Read the model definition and answer for the solid it produces. Units are mm, in the model's axes. Coordinates: 2 decimals unless noted, no trailing zeros. Loops run counter-clockwise (first coordinate to the right, second up) from the corner with the lowest first, then second, coordinate; pieces in that order, holes last. Notation, with made-up numbers: M 24.25,18.25 L 30.25,18.25 A22 cw 30.25,37.25 Z; hole C 27.25,-0.5 d11. An arc over 180 degrees is marked long. One line per item, written item: value. Start each with the question number.
1. The part is cut by section C-C (y = -21.5). Write down the section's boundary in (x, z).
2. Determine the mould class of faces 1 (the face through (-16, -41, 0)), 2 (the face through (-14.276, 47, 3)), 3 (the face through (-1, -62.803, 3)), 4 (the face through (-56.78, 56.76, 3.22)) for opening direction Y: +Y half, -Y half, draft (parallel to the pull), parting line (faces both ways), or undercut.
3. A flat-ended cylindrical pin translates along its axis: pin 1 (6.5 mm diameter, centred on x = -55.9, y = -53.99, fed in from +Z). Find the tip coordinate at first contact, or state that the pin passes through.
4. The part is cut by section D-D (z = 4.5). State how many separate pieces and enclosed holes the cut face has, then the cut area to 3 significant figures.
5. Consider probe 1 along Y at (x, z) = (57, 2); probe 2 along X at (y, z) = (-16.5, 0.5); probe 3 along Y at (x, z) = (-4.5, 3.75). Determine where each line is inside the solid, lowest interval first.
6. The part is cut by section A-A (x = 27). Write down the section's boundary in (y, z), then the cut area to 3 significant figures.
7. The part is cut by section B-B (x = 58). Write down the section's boundary in (y, z), then the cut area to 3 significant figures.
```python
from build123d import *

# Parameters (mm, degrees)
SKETCH2_W           = 132.7
SKETCH2_H           = 125
BOSS_EXTRUDE1_DEPTH = 6.35
SKETCH1_R           = 2
CUT_EXTRUDE1_DEPTH  = 6.35
SKETCH6_R           = 4
CUT_EXTRUDE3_DEPTH  = 6.35


with BuildPart() as part:
    # Sketch2 → Boss-Extrude1 (new body)
    with BuildSketch(Plane.XY):
        with Locations((-0.075710713, -0.302842853)):
            Rectangle(SKETCH2_W, SKETCH2_H)
    extrude(amount=BOSS_EXTRUDE1_DEPTH)

    # Sketch1 → Cut-Extrude1 (cut)
    with BuildSketch(Plane.XY):
        with Locations(Location((-50.481706077, 16.075057848, 0), (0, 0, 180))):
            Circle(SKETCH1_R)
        with Locations(Location((-50.481706077, -16.680743555, 0), (0, 0, 180))):
            Circle(SKETCH1_R)
        with Locations(Location((-31.228329085, -43.180743555, 0), (0, 0, 180))):
            Circle(SKETCH1_R)
        with Locations(Location((-0.075710713, -53.302842853, 0), (0, 0, 180))):
            Circle(SKETCH1_R)
        with Locations(Location((31.076907658, -43.180743555, 0), (0, 0, 180))):
            Circle(SKETCH1_R)
        with Locations(Location((50.33028465, -16.680743555, 0), (0, 0, 180))):
            Circle(SKETCH1_R)
        with Locations(Location((50.33028465, 16.075057848, 0), (0, 0, 180))):
            Circle(SKETCH1_R)
        with Locations(Location((31.076907658, 42.575057848, 0), (0, 0, 180))):
            Circle(SKETCH1_R)
        with Locations(Location((-31.228329085, 42.575057848, 0), (0, 0, 180))):
            Circle(SKETCH1_R)
        with BuildLine():
            Line((-14.275710713, 39.754740698), (-14.275710713, 54.754740698))
            Line((-14.275710713, 54.754740698), (14.124289287, 54.754740698))
            Line((14.124289287, 54.754740698), (14.124289287, 39.754740698))
            ThreePointArc((14.124289287, 39.754740698), (-0.075710713, -42.802842853), (-14.275710713, 39.754740698))
        make_face()
    extrude(amount=CUT_EXTRUDE1_DEPTH, mode=Mode.SUBTRACT)

    # Sketch6 → Cut-Extrude3 (cut)
    with BuildSketch(Plane.XY.offset(6.35)):
        with Locations((58.774289287, -53.990342854)):
            Circle(SKETCH6_R)
        with Locations((43.774289287, -53.990342854)):
            Circle(SKETCH6_R)
        with Locations((-55.903321393, -53.990342853)):
            Circle(SKETCH6_R)
        with Locations((-43.403321393, -53.990342853)):
            Circle(SKETCH6_R)
        with Locations((-58.925710713, 53.384657146)):
            Circle(SKETCH6_R)
        with Locations((-43.925710713, 53.384657146)):
            Circle(SKETCH6_R)
        with Locations((43.774289287, 53.384657147)):
            Circle(SKETCH6_R)
        with Locations((58.774289287, 53.384657147)):
            Circle(SKETCH6_R)
    extrude(amount=-CUT_EXTRUDE3_DEPTH, mode=Mode.SUBTRACT)


solid = part.part
```
Answer block:
1. outline: M -66.43,0 L -36.91,0 L -36.91,6.35 L -66.43,6.35 Z; M 36.76,0 L 66.27,0 L 66.27,6.35 L 36.76,6.35 Z
2. face 1: draft
2. face 2: undercut
2. face 3: -Y half
2. face 4: undercut
3. pin 1: passes through
4. separate pieces: 1
4. enclosed holes: 18
4. area: 10,000 mm2
5. probe 1: y = -62.8 to -57.58, -50.41 to 49.8, 56.97 to 62.2
5. probe 2: x = -66.43 to -52.47, -48.49 to -39.37, 39.22 to 48.34, 52.32 to 66.27
5. probe 3: y = -62.8 to -42.57, 54.75 to 62.2
6. outline: M -62.8,0 L -33.06,0 L -33.06,6.35 L -62.8,6.35 Z; M 32.46,0 L 62.2,0 L 62.2,6.35 L 32.46,6.35 Z
6. area: 378 mm2
7. outline: M -62.8,0 L -57.91,0 L -57.91,6.35 L -62.8,6.35 Z; M -50.07,0 L 49.46,0 L 49.46,6.35 L -50.07,6.35 Z; M 57.31,0 L 62.2,0 L 62.2,6.35 L 57.31,6.35 Z
7. area: 694 mm2
